Geometry: final body of the model. Coordinates: model frame, mm. Face numbers are marked on the shaded views. A direction names the side the tool comes from. Coordinates: 2 decimals unless noted, no trailing zeros. Order: outer loops, then holes, each group sorted by start corner. A loop starts at its lowest first (then second) coordinate and runs counter-clockwise, first axis right, second up. Notation, with made-up numbers: M -26.75,30.25 L -15.75,30.25 A25 ccw -15.75,65.25 Z; hole C 73.5,34.5 d2. An arc over 180 degrees is marked long. One line per question, with ' | ' between items.
from build123d import *


with BuildPart() as part:
    # Sketch1 → Revolve2 (revolve)
    with BuildSketch(Plane(origin=(0, 0, 0), x_dir=(0, 0, -1), z_dir=(1, 0, 0)), mode=Mode.PRIVATE) as revolve2_sk:
        Polygon((-25.4, 12.7), (25.4, 12.7), (25.4, 22.225), (3.175, 22.225), (3.175, 63.5), (19.05, 63.5), (19.05, 88.9), (-19.05, 88.9), (-19.05, 63.5), (-3.175, 63.5), (-3.175, 22.225), (-25.4, 22.225), align=None)
    revolve(revolve2_sk.sketch.rotate(Axis((0, 0, 0), (0, 0, -1)), 90), axis=Axis((0, 0, 0), (0, 0, -1)))

    # Sketch2 → Cut-Revolve1 (revolve, cut)
    with BuildSketch(Plane(origin=(0, 0, 0), x_dir=(0, 0, -1), z_dir=(1, 0, 0)), mode=Mode.PRIVATE) as cut_revolve1_sk:
        Polygon((-10.972421975, 88.687029024), (-6.35, 75.987029024), (6.35, 75.987029024), (10.972421975, 88.687029024), align=None)
    revolve(cut_revolve1_sk.sketch.rotate(Axis((0, 0, 0), (0, 0, -1)), 90), axis=Axis((0, 0, 0), (0, 0, -1)), mode=Mode.SUBTRACT)


solid = part.part
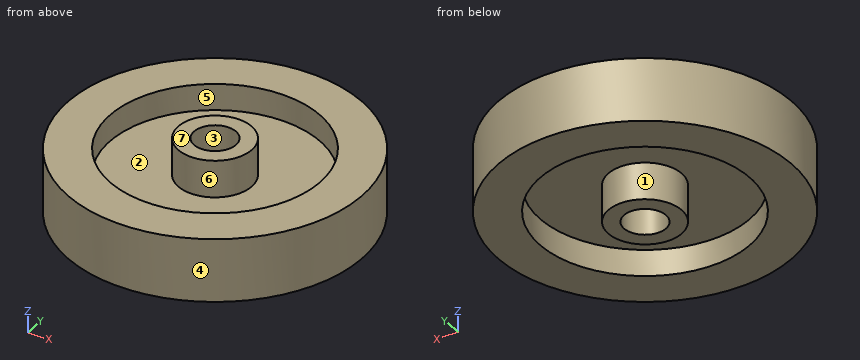
1. Access query for the marked faces 1, 2 and 3. Directions: +Z, -Z, +X, -X, +Y, -Y. A direction counts if a zero-diameter tool reaches every point of the face in a straight line with its end or side. Return the directions, or none.
Response values:
face 1: -Z | face 2: +Z | face 3: +Z, -Z
2. Material intervals for line 1 (Y direction, x = 0, z = -14) (3 decimals); line 2 (Y direction, x = 0, z = 2.25); line 3 (X direction, y = -7, z = 4), sorted ascending. Write a range as [from, to].
Response values:
line 1: y = [-88.9, -63.5], [-22.225, -12.7], [12.7, 22.225], [63.5, 88.9] | line 2: y = [-88.9, -88.69], [-75.99, -12.7], [12.7, 75.99], [88.69, 88.9] | line 3: x = [-88.62, -88.41], [-75.66, -63.11], [-21.09, -10.6], [10.6, 21.09], [63.11, 75.66], [88.41, 88.62]
3. Section A-A, the plane y = 0. Give the number of separate pieces and of enclosed holes in the cut face, and give its area (3 significant figures).
Response values:
separate pieces: 2 | enclosed holes: 2 | area: 2,990 mm^2
4. Section C-C, the plane z = -1. Output: boundary loops of the cut face in (x, y), and give its area (3 significant figures).
Response values:
outline: C 0,0 d177.8; C 0,0 d151.97; hole C 0,0 d177.37; hole C 0,0 d25.4 | area: 17,800 mm^2
5. Pin query (flat end, axial travel): P1, Ø10, axis at x = -61, y = 67, coming from the -Z side; P2, Ø6, axis at y = 18, z = -9.5, coming from the +X side; P3, Ø1.5, axis at x = -2.5, y = -26.5, coming from the -Z side (3 decimals); P4, Ø1.5, axis at x = 45, z = -20.5, coming from the +Y side. Return the tip coordinate at first contact, or that it passes through.
Response values:
P1: stops at z = -19.05 | P2: stops at x = 87.63 | P3: stops at z = -3.175 | P4: passes through
6. Draft query along X for the marked faces 4, 5, 6 and 7. Return one class per face: pulls with the +X half, pulls with the -X half, needs draft (parallel to the pull), parting line crosses it, or undercut.
Response values:
face 4: parting line crosses it | face 5: undercut | face 6: undercut | face 7: needs draft
